```python
from build123d import *

# Parameters (mm, degrees)
BOSS_EXTRUDE1_DEPTH = 100.5
TAP1_D              = 4.134
TAP1_DEPTH          = 12.4
TAP1_TIP            = 1.2419789
TAP2_D              = 4.134
TAP2_DEPTH          = 12.4
TAP2_TIP            = 1.2419789


with BuildPart() as part:
    # Sketch1 → Boss-Extrude1 (new body)
    with BuildSketch(Plane(origin=(0, 0, 0), x_dir=(0, 0, -1), z_dir=(1, 0, 0))):
        Polygon((0, -4.618802154), (4, -2.309401077), (4, 2.309401077), (0, 4.618802154), (-4, 2.309401077), (-4, -2.309401077), align=None)
    extrude(amount=BOSS_EXTRUDE1_DEPTH)

    # Sketch2 → Cut-Revolve1 (revolve, cut)
    with BuildSketch(Plane.XY):
        Polygon((0, 4.618802154), (0.35726559, 4.618802154), (0, 4), align=None)
        Polygon((100.14273441, 4.618802154), (100.5, 4), (100.5, 4.618802154), align=None)
    revolve(axis=Axis((0, 0, 0), (1, 0, 0)), mode=Mode.SUBTRACT)

    # Tap1
    with Locations(Plane.ZY):
        with Locations((0, 0)):
            Hole(TAP1_D / 2, depth=TAP1_DEPTH)
            with Locations((0, 0, -(TAP1_DEPTH + TAP1_TIP / 2))):  # 118° drill point
                Cone(0, TAP1_D / 2, TAP1_TIP, mode=Mode.SUBTRACT)

    # Tap2
    with Locations(Plane(origin=(100.5, 0, 0), x_dir=(0, 0, -1), z_dir=(1, 0, 0))):
        with Locations((0, 0)):
            Hole(TAP2_D / 2, depth=TAP2_DEPTH)
            with Locations((0, 0, -(TAP2_DEPTH + TAP2_TIP / 2))):  # 118° drill point
                Cone(0, TAP2_D / 2, TAP2_TIP, mode=Mode.SUBTRACT)


solid = part.part
```
Could you check a few things on this model? Use its own coordinates, in mm. A direction names the side the tool comes from. Give positions to 0.01 mm unless a question says otherwise; leave off trailing zeros. Write each loop counter-clockwise with the first axis right and the second up, starting at its lowest first coordinate (ties: lowest second). Pieces come first, ordered by that corner, then holes. Notation, with made-up numbers: (24.25, 4) - (67.25, 4) arc R16 ccw to (67.25, 19) - close; hole circle Ø2 at (58, 10.5). An arc over 180 degrees is marked (long way). One line per item, written item: value. Start each with the question number.
Item 1: Imagine slicing it at A-A, the plane x = 43. List the corners of the cut face in (y, z) for me.
Item 2: Which directions (+Z, -Z, +X, -X, +Y, -Y) give clear straight access to the entire face, cutting with the end or side of a thin tool? Please do faces 4 (the face through (94.21, -1.26, -1.64)), 5 (the face through (0.085, -2.065, 3.597)).
Item 3: I'm going to push flat-ended pins straight in: pin 1 (2.5 mm diameter, centred on y = 0, z = 0, fed in from +X); pin 2 (3 mm diameter, centred on x = 83, z = 2.5, fed in from +Y). Where does each tip first touch, or does it pass through?
Item 4: If we mould it in two halves opening along Z, with no side actions, what happens to faces 1 (the face through (49.547, -3.448, 2.028)), 2 (the face through (49.547, 3.448, -2.028)), 3 (the face through (87.074, -0.35, 0.078))? For each: +Z half, -Z half, draft (parallel to the pull), parting line (faces both ways), or undercut.
Item 5: Please list where these lines run through material, in increasing order: line 1 (Y direction, x = 92.25, z = 0); line 2 (Z direction, x = 92, y = 0); line 3 (Y direction, x = 57, z = 2). Write a range as from..to.
Geometry says:
1. outline: (-4.62, 0) - (-2.31, -4) - (2.31, -4) - (4.62, 0) - (2.31, 4) - (-2.31, 4) - close
2. face 4: +X
2. face 5: +Z, -X, -Y
3. pin 1: x = 87.61
3. pin 2: y = 4.04
4. face 1: +Z half
4. face 2: -Z half
4. face 3: undercut
5. line 1: -4.62..-2.07, 2.07..4.62
5. line 2: -4..-2.07, 2.07..4
5. line 3: -3.46..3.46
